from build123d import *

# Parameters (mm, degrees)
SKETCH1_R           = 1.598426077
SKETCH1_R_2         = 3
BOSS_EXTRUDE1_DEPTH = 2
SCALE1_SCALE        = 2.8


with BuildPart() as part:
    # Sketch1 → Boss-Extrude1 (new body)
    with BuildSketch(Plane.XY):
        with BuildLine():
            Line((-185.215931952, 133.947260869), (-185.213664396, 133.947234502))
            Line((-185.213664396, 133.947234502), (-181.222608058, 134.40739012))
            add(Edge.make_bspline(
                [(-181.222608058, 134.40739012), (-179.470077492, 134.609439885), (-178.007424926, 135.082040692), (-176.58956977, 134.02354039)],
                knots=[0.1, 0.1, 0.1, 0.1, 0.133333333, 0.133333333, 0.133333333, 0.133333333], degree=3))
            add(Edge.make_bspline(
                [(-176.58956977, 134.02354039), (-175.053406211, 132.876684515), (-173.674389539, 130.527654949), (-173.900512309, 130.490108445)],
                knots=[0.133333333, 0.133333333, 0.133333333, 0.133333333, 0.166666667, 0.166666667, 0.166666667, 0.166666667], degree=3))
            Line((-173.900512309, 130.490108445), (-184.336884958, 128.757089405))
            Line((-184.336884958, 128.757089405), (-184.173119971, 127.817925817))
            Line((-184.173119971, 127.817925817), (-192.016779912, 126.651189278))
            add(Edge.make_bspline(
                [(-192.016779912, 126.651189278), (-192.907955692, 126.552708804), (-193.71626022, 126.739571219), (-194.466926644, 127.127560556)],
                knots=[0.266666667, 0.266666667, 0.266666667, 0.266666667, 0.3, 0.3, 0.3, 0.3], degree=3))
            Line((-194.466926644, 127.127560556), (-195.306587773, 127.817925817))
            Line((-195.306587773, 127.817925817), (-212.023872072, 123.761509934))
            ThreePointArc((-212.023872072, 123.761509934), (-217.37856884, 127.123951805), (-213.87424985, 132.386892164))
            Line((-213.87424985, 132.386892164), (-208.863883058, 133.322461629))
            Line((-208.863883058, 133.322461629), (-206.408455346, 132.448142845))
            Line((-206.408455346, 132.448142845), (-198.430956882, 134.26057907))
            add(Edge.make_bspline(
                [(-198.430956882, 134.26057907), (-196.41657636, 134.684664731), (-195.322164303, 134.996216346), (-194.244996216, 134.835931794)],
                knots=[0.833333333, 0.833333333, 0.833333333, 0.833333333, 0.866666667, 0.866666667, 0.866666667, 0.866666667], degree=3))
            add(Edge.make_bspline(
                [(-194.244996216, 134.835931794), (-193.666057591, 134.749817409), (-193.283526207, 134.691889269), (-192.335160561, 134.072002805)],
                knots=[0.866666667, 0.866666667, 0.866666667, 0.866666667, 0.9, 0.9, 0.9, 0.9], degree=3))
            ThreePointArc((-192.335160561, 134.072002805), (-188.713175288, 137.569246142), (-185.215931952, 133.947260869))
        make_face()
        with Locations((-213.064337356, 128.049471145)):
            Circle(SKETCH1_R, mode=Mode.SUBTRACT)
        with Locations((-188.775546256, 134.009631837)):
            Circle(SKETCH1_R_2, mode=Mode.SUBTRACT)
    extrude(amount=BOSS_EXTRUDE1_DEPTH)


with BuildPart() as part_1:
    # Scale1: scaled about (-197.812909455, 130.051467898, 1)
    add(part.part.scale(SCALE1_SCALE).moved(Location((356.063237019, -234.092642216, -1.8))))


solid = part_1.part
For this review, take the finished solid that the model builds, in its own axes (mm). A direction names the side the tool comes from. Give positions to 0.01 mm unless a question says otherwise; leave off trailing zeros. Order: outer loops, then holes, each group sorted by start corner. A loop starts at its lowest first (then second) coordinate and runs counter-clockwise, first axis right, second up. Notation, with made-up numbers: (-9.75, 48.25) - (17.25, 48.25) arc R16 ccw to (17.25, 64.25) - close; hole circle Ø3 at (41, 77). An arc over 180 degrees is marked (long way). Answer as a JSON object with one key per item and string values. Group by question number.
Item 1: Clearance check with flat-ended pins moving along their axes: pin 1 Ø6 at (x, y) = (-170.5, 122) entering from -Z; pin 2 Ø1.5 at (x, z) = (-189.5, 2) entering from +Y; pin 3 Ø2 at (y, z) = (120.5, 2.5) entering from -X; pin 4 Ø2 at (x, z) = (-175, 2) entering from +Y. State where each tip first meets the part, or that it passes through.
Item 2: Draft analysis for pull direction X (two halves, no side actions). For faces 1 (the flat face through (-204, 132, 3.8)), 2 (the flat face through (-210.868, 139.264, 0.961)), 3 (the flat face through (-159.854, 125.131, 0.961)), state which applies: pulls with the +X half, pulls with the -X half, needs draft (parallel to the pull), parting line crosses it, or undercut.
Item 3: Machinability: for faces 4 (the cylindrical face through (-238.452, 120.475, 0.961)), 5 (the flat face through (-157.026, 141.595, 0.961)), 6 (the flat face through (-213.87, 118.2, 0.96)), which of the approach directions +Z, -Z, +X, -X, +Y, -Y give a long, thin tool a straight path to every point of the face, cutting with its end or side? Answer none if there is none.
Item 4: Wall thickness on line 1 along Y through (x, z) = (-179, 0.05); line 2 along Y through (x, z) = (-237, 0.1); line 3 along X through (y, z) = (124.5, 0.25): over which ranges is each line inside the solid? List them lowest first.
Item 5: Take a section at A-A on y = 145.5. Give the boundary of the cut face in (x, z), and give its area (3 significant figures).
Item 6: Take a section at D-D on z = 2.5. Give the number of separate pieces and of enclosed holes in the cut face, and give its area (3 significant figures).
Item 7: Take a section at B-B on x = -207.5. Give the boundary of the cut face in (y, z).
Item 8: Take a section at C-C on y = 116. Give the boundary of the cut face in (x, z).
Reported:
{
 "1": {"pin 1": "z = -1.8", "pin 2": "y = 143.57", "pin 3": "x = -252.52", "pin 4": "y = 150.99"},
 "2": {"face 1": "needs draft", "face 2": "undercut", "face 3": "pulls with the +X half"},
 "3": {"face 4": "+Z, -Z", "face 5": "+Z, -Z, +Y", "face 6": "+Z, -Z, -Y"},
 "4": {"line 1": "120.92 to 135.8, 146.47 to 148.7", "line 2": "112.59 to 121.68, 127.21 to 137.67", "line 3": "-252.87 to -244.99, -236.04 to -159.74"},
 "5": {"outline": "(-181.47, -1.8) - (-179.68, -1.8) - (-179.68, 3.8) - (-181.47, 3.8) - close; (-165.33, -1.8) - (-163.55, -1.8) - (-163.55, 3.8) - (-165.33, 3.8) - close", "area": "20.0 mm^2"},
 "6": {"separate pieces": "1", "enclosed holes": "2", "area": "2,150 mm^2"},
 "7": {"outline": "(119.74, -1.8) - (140.03, -1.8) - (140.03, 3.8) - (119.74, 3.8) - close"},
 "8": {"outline": "(-249.53, -1.8) - (-222.93, -1.8) - (-222.93, 3.8) - (-249.53, 3.8) - close"}
}
